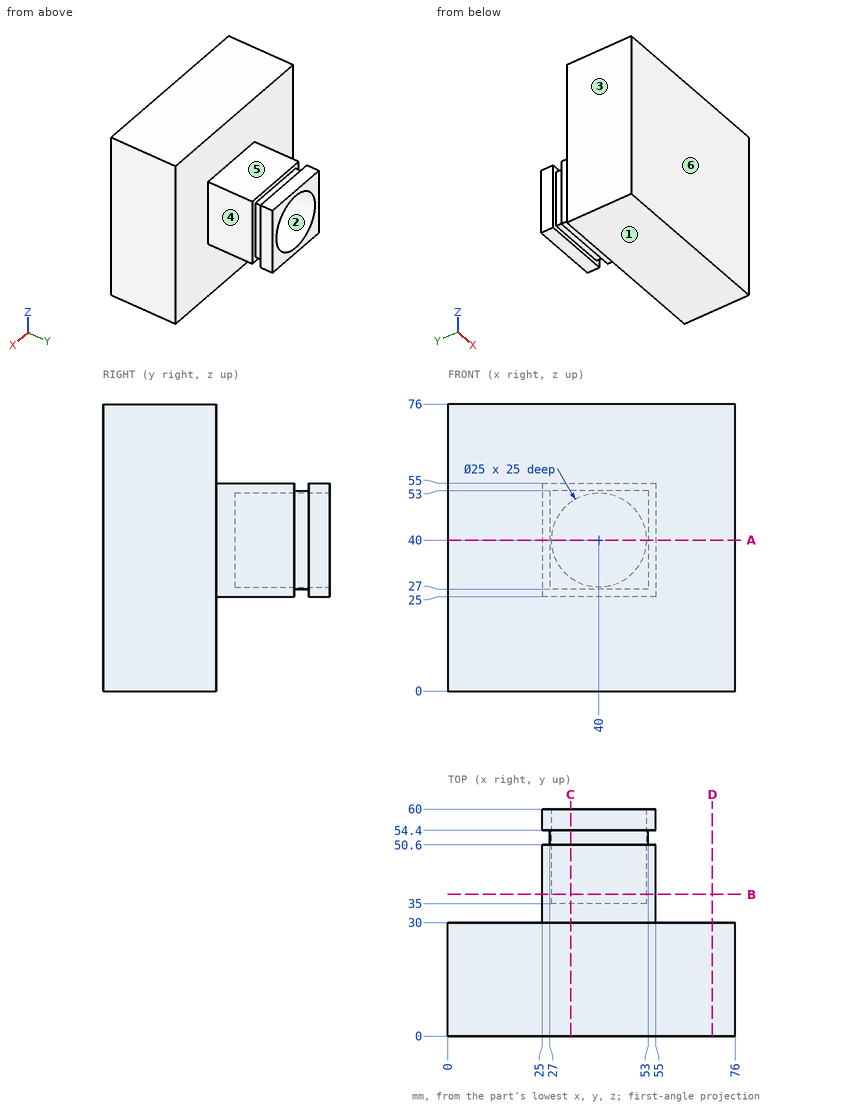
For this review, use the dimensioned drawing (mm, ordinates from the lowest corner) and the shaded views. A direction names the side the tool comes from. Coordinates: 2 decimals unless noted, no trailing zeros. Loops run counter-clockwise (first coordinate to the right, second up) from the corner with the lowest first, then second, coordinate; pieces in that order, holes last. Notation, with made-up numbers: (47, 79) - (61, 79) arc R16 cw to (61, 90) - close; hole circle Ø5 at (64, 79). An arc over 180 degrees is marked (long way). Use CSV: the item, a comma, the result in double quotes. Start each with the question number.
1) Consider section D-D on x = 70. Write out the cut boundary in (y, z), then the cut area to 3 significant figures.
2) Wall thickness on L1, parallel to X at y = 53, z = 40; L2, parallel to Y at x = 32, z = 54; L3, parallel to Z at x = 40, y = 46.75: over which ranges is each line inside the solid? List them lowest first. Write a range as from..to.
3) Consider section C-C on x = 32.5. Write out the cut boundary in (y, z), then the cut area to 3 significant figures.
4) Tool access review of the marked faces 4, 5 and 6: name each direction out of +Z, -Z, +X, -X, +Y, -Y from which nothing blocks a thin tool from reaching the whole face with its end or side.
5) For pin 1 Ø1 at (x, z) = (17, 52) entering from -Y; pin 2 Ø4.5 at (y, z) = (56, 38) entering from +X; pin 3 Ø6 at (x, y) = (46.5, 56.5) entering from +Z; pin 4 Ø3 at (x, y) = (54.5, 49.5) entering from -Z, all flat-tipped, find the tip position at first contact; note any pin that passes through.
6) Consider section A-A on z = 40. Write out the cut boundary in (x, y), then the cut area to 3 significant figures.
7) The part is to be moulded in two halves that separate along Z. For the marked faces 1, 2 and 3, say which applies: +Z half, -Z half, draft (parallel to the pull), parting line (faces both ways), or undercut.
8) Consider section B-B on y = 37.5. Write out the cut boundary in (x, z), then the cut area to 3 significant figures.
Geometry says:
1,outline,"(0, 0) - (30, 0) - (30, 76) - (0, 76) - close"
1,area,"2,280 mm^2"
2,L1,"27..27.5, 52.5..53"
2,L2,"0..50.6, 54.4..60"
2,L3,"25..27.5, 52.5..55"
3,outline,"(0, 0) - (30, 0) - (30, 25) - (50.6, 25) - (50.6, 27) - (54.4, 27) - (54.4, 25) - (60, 25) - (60, 30) - (35, 30) - (35, 50) - (60, 50) - (60, 55) - (54.4, 55) - (54.4, 53) - (50.6, 53) - (50.6, 55) - (30, 55) - (30, 76) - (0, 76) - close"
3,area,"2,660 mm^2"
4,face 4,"+Z, -Z, +X, +Y"
4,face 5,"+Z, +X, -X, +Y"
4,face 6,"+Z, -Z, +X, -X, -Y"
5,pin 1,"y = 0"
5,pin 2,"x = 55"
5,pin 3,"z = 55"
5,pin 4,"z = 25"
6,outline,"(0, 0) - (76, 0) - (76, 30) - (55, 30) - (55, 50.6) - (53, 50.6) - (53, 54.4) - (55, 54.4) - (55, 60) - (52.5, 60) - (52.5, 35) - (27.5, 35) - (27.5, 60) - (25, 60) - (25, 54.4) - (27, 54.4) - (27, 50.6) - (25, 50.6) - (25, 30) - (0, 30) - close"
6,area,"2,540 mm^2"
7,face 1,"-Z half"
7,face 2,"undercut"
7,face 3,"draft"
8,outline,"(25, 25) - (55, 25) - (55, 55) - (25, 55) - close; hole circle Ø25 at (40, 40)"
8,area,"409 mm^2"
